For this review, take the finished solid that the model builds, in its own axes (mm). A direction names the side the tool comes from. Give positions to 0.01 mm unless a question says otherwise; leave off trailing zeros. Order: outer loops, then holes, each group sorted by start corner. A loop starts at its lowest first (then second) coordinate and runs counter-clockwise, first axis right, second up. Notation, with made-up numbers: (-13.5, 41) - (41.5, 41) arc R30 cw to (41.5, 71) - close; hole circle Ø3 at (75, 17.5). An arc over 180 degrees is marked (long way). Use a Markdown table: item, result. Add a question column.
1) Clearance check with flat-ended pins moving along their axes: P1, Ø0.7, axis at y = 9.5, z = 0.5, coming from the -X side; P2, Ø1.6, axis at x = 2, z = -0.5, coming from the -Y side; P3, Ø1.2, axis at x = -1.5, z = 1, coming from the -Y side. State where each tip first meets the part, or that it passes through.
2) Wall thickness on L1, parallel to Y at x = 0, z = 1.75; L2, parallel to Y at x = 0, z = -0.5; L3, parallel to X at y = 0, z = -0.4: over which ranges is each line inside the solid? List them lowest first.
3) We need section D-D on z = -0.65. Give the number of separate pieces and of enclosed holes in the cut face, then the cut area to 3 significant figures.
4) Mouldability with a two-part tool opening along Y and no side actions: class faces 4 (the face through (-1.76, -4.86, 0.03)), 5 (the face through (0.1, 11.6, 0)), 6 (the face through (-2, -7.2, 0)), 7 (the face through (-3, 3, -2)) as released by +Y, released by -Y, zero draft, split by the parting line, or undercut.
5) Machinability: for faces 1 (the face through (2, -2, 1.2)), 2 (the face through (-3.6, 0, 0)), 3 (the face through (0, -10.4, 0)), which of the approach directions +Z, -Z, +X, -X, +Y, -Y give a long, thin tool a straight path to every point of the face, cutting with its end or side? Answer none if there is none.
6) We need section A-A on y = -6.5. Write out the cut boundary in (x, z).
7) We need section C-C on y = 0. Write out the cut boundary in (x, z).
8) We need section B-B on x = 0. Write out the cut boundary in (y, z), then the cut area to 3 significant figures.
Autodesk Inventor part; units mm, degrees
ref_plane "YZ Plane" through (0, 0, 0) normal (1, 0, 0) x (0, 1, 0)
ref_plane "XZ Plane" through (0, 0, 0) normal (0, 1, 0) x (-1, 0, 0)
ref_plane "XY Plane" through (0, 0, 0) normal (0, 0, 1) x (1, 0, 0)
sketch "Sketch1" plane through (0, 0, 0) normal (0, 0, 1) x (1, 0, 0)
  line L0 (3.6, -8) -> (3.6, 8)
  line L1 (-3.6, 8) -> (-3.6, -8)
  arc A0 (3.6, 8) -> (-3.6, 8) centre (0, 8) ccw
  circle A1 centre (0, 8) radius 2.4 construction
  circle A2 centre (0, 8) radius 3.2 construction
  circle A3 centre (0, 0) radius 3.2
  circle A4 centre (0, 0) radius 2.4
  line L2 (0, 0) -> (0, 8) construction
  line L3 (-2.8, 5.7373) -> (-2.8, 2.2627)
  line L4 (2.8, 5.7373) -> (2.8, 2.2627)
  arc A5 (-2.8, 5.7373) -> (2.8, 5.7373) centre (0, 8) ccw
  arc A6 (2.8, 2.2627) -> (-2.8, 2.2627) centre (0, 0) ccw
  arc A7 (-3.6, -8) -> (3.6, -8) centre (0, -8) ccw
  circle A8 centre (0, -8) radius 3.2 construction
  circle A9 centre (0, -8) radius 2.4 construction
  line L5 (0, 0) -> (0, -8) construction
  line L6 (-2.8, -2.2627) -> (-2.8, -5.7373)
  line L7 (2.8, -2.2627) -> (2.8, -5.7373)
  arc A10 (-2.8, -2.2627) -> (2.8, -2.2627) centre (0, 0) ccw
  arc A11 (2.8, -5.7373) -> (-2.8, -5.7373) centre (0, -8) ccw
  line L8 (0.8, 4.49) -> (0.8, 7.2)
  line L9 (0.8, 7.2) -> (2.2627, 7.2)
  line L10 (2.2627, 8.8) -> (0.8, 8.8)
  line L11 (0.8, 8.8) -> (0.8, 10.2627)
  line L12 (-0.8, 10.2627) -> (-0.8, 8.8)
  line L13 (-0.8, 8.8) -> (-2.2627, 8.8)
  line L14 (-2.2627, 7.2) -> (-0.8, 7.2)
  line L15 (-0.8, 7.2) -> (-0.8, 4.49)
  arc A12 (-2.2627, 8.8) -> (-2.2627, 7.2) centre (0, 8) ccw
  arc A13 (0.8, 10.2627) -> (-0.8, 10.2627) centre (0, 8) ccw
  arc A14 (2.2627, 7.2) -> (2.2627, 8.8) centre (0, 8) ccw
  line L16 (-0.8, -10.2627) -> (-0.8, -8.8)
  line L17 (-0.8, -8.8) -> (-2.2627, -8.8)
  line L18 (-2.2627, -7.2) -> (-0.8, -7.2)
  line L19 (-0.8, -7.2) -> (-0.8, -4.49)
  line L20 (0.8, -4.49) -> (0.8, -7.2)
  line L21 (0.8, -7.2) -> (2.2627, -7.2)
  line L22 (2.2627, -8.8) -> (0.8, -8.8)
  line L23 (0.8, -8.8) -> (0.8, -10.2627)
  arc A15 (-2.2627, -7.2) -> (-2.2627, -8.8) centre (0, -8) ccw
  arc A16 (-0.8, -10.2627) -> (0.8, -10.2627) centre (0, -8) ccw
  arc A17 (2.2627, -8.8) -> (2.2627, -7.2) centre (0, -8) ccw
  dimension "d8" = 4.8
  dimension "d9" = 6.4
  dimension "d32" = 7.2
  dimension "d34" = 8
  dimension "d36" = 0.8
  dimension "d52" = 1.6
extrude "Extrusion1" add sketch "Sketch1" along normal mid plane 4 contours A7 L1 A0 L0 | A3
sketch "Sketch6" plane through (0, 0, 2) normal (0, 0, 1) x (1, 0, 0)
  circle A0 centre (0, 0) radius 3.1
  circle A1 centre (0, 0) radius 2.4
  dimension "d53" = 6.2
extrude "Extrusion7" cut sketch "Sketch6" against normal blind 0.8 contours A0 | A1
mirror "Mirror1" about plane through (0, 0, 0) normal (0, 0, 1) of "Extrusion7"
fillet "Fillet1" radius 0.1 6 edges at (0, 11.6, 2) (3.6, 0, 2) (-3.6, 0, 2) (0, 11.6, -2) (-3.6, 0, -2) (3.6, 0, -2)
fillet "Fillet1" radius 0.4 12 edges at (-2.8, -2.2627, 0) (-2.8, -5.7373, 0) (2.8, -5.7373, 0) (2.8, -2.2627, 0) (-2.8, 5.7373, 0) (-2.8, 2.2627, 0) (-0.8, -4.49, 0) (0.8, -4.49, 0) (2.8, 2.2627, 0) (2.8, 5.7373, 0) (0.8, 4.49, 0) (-0.8, 4.49, 0)
equation "\"d8\" = kd"
equation "\"d9\" = tsd"
equation "\"d32\" = tlad"
equation "\"d34\" = lu"
equation "\"d52\" = axlet"
equation "\"d14\" = 0.5 * lu"
equation "\"d41\" = tsl"
equation "\"d45\" = lf"
equation "\"d46\" = tf"
properties part number "6632-LtBluishGray" material "ABS Plastic"
Checked values:
| question | item | result |
|---|---|---|
| 1 | P1 | x = -3.41 |
| 1 | P2 | y = -11.39 |
| 1 | P3 | y = -11.49 |
| 2 | L1 | -11.6 to -10.4, -3.6 to -3.1, 3.1 to 3.6, 10.4 to 11.6 |
| 2 | L2 | -11.6 to -10.4, -3.6 to -2.4, 2.4 to 3.6, 10.4 to 11.6 |
| 2 | L3 | -3.6 to -2.4, 2.4 to 3.6 |
| 3 | separate pieces | 1 |
| 3 | enclosed holes | 3 |
| 3 | area | 91.9 mm² |
| 4 | face 4 | undercut |
| 4 | face 5 | released by +Y |
| 4 | face 6 | undercut |
| 4 | face 7 | zero draft |
| 5 | face 1 | +Z |
| 5 | face 2 | +Z, -Z, -X, +Y, -Y |
| 5 | face 3 | +Z, -Z |
| 6 | outline | (-3.6, -1.9) arc R0.1 ccw to (-3.5, -2) - (-0.8, -2) - (-0.8, 2) - (-3.5, 2) arc R0.1 ccw to (-3.6, 1.9) - close; (0.8, -2) - (3.5, -2) arc R0.1 ccw to (3.6, -1.9) - (3.6, 1.9) arc R0.1 ccw to (3.5, 2) - (0.8, 2) - close |
| 7 | outline | (-3.6, -1.9) arc R0.1 ccw to (-3.5, -2) - (-3.1, -2) - (-3.1, -1.2) - (-2.4, -1.2) - (-2.4, 1.2) - (-3.1, 1.2) - (-3.1, 2) - (-3.5, 2) arc R0.1 ccw to (-3.6, 1.9) - close; (2.4, -1.2) - (3.1, -1.2) - (3.1, -2) - (3.5, -2) arc R0.1 ccw to (3.6, -1.9) - (3.6, 1.9) arc R0.1 ccw to (3.5, 2) - (3.1, 2) - (3.1, 1.2) - (2.4, 1.2) - close |
| 8 | outline | (-11.6, -1.9) arc R0.1 ccw to (-11.5, -2) - (-10.4, -2) - (-10.4, 2) - (-11.5, 2) arc R0.1 ccw to (-11.6, 1.9) - close; (-3.6, -2) - (-3.1, -2) - (-3.1, -1.2) - (-2.4, -1.2) - (-2.4, 1.2) - (-3.1, 1.2) - (-3.1, 2) - (-3.6, 2) - close; (2.4, -1.2) - (3.1, -1.2) - (3.1, -2) - (3.6, -2) - (3.6, 2) - (3.1, 2) - (3.1, 1.2) - (2.4, 1.2) - close; (10.4, -2) - (11.5, -2) arc R0.1 ccw to (11.6, -1.9) - (11.6, 1.9) arc R0.1 ccw to (11.5, 2) - (10.4, 2) - close |
| 8 | area | 17.0 mm² |
